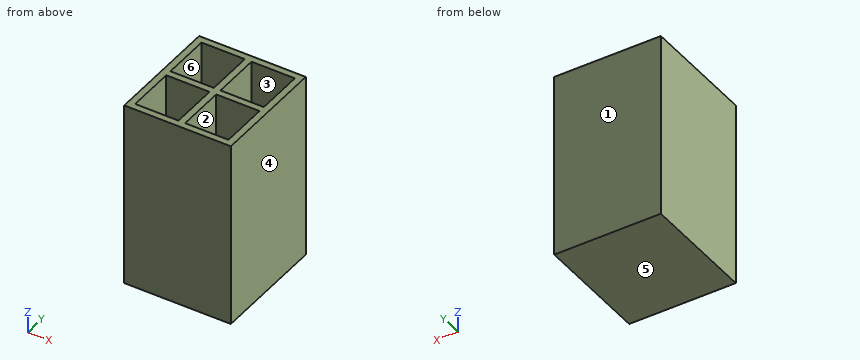
from build123d import *

# Parameters (mm, degrees)
F0_W     = 50.931696
F0_H     = 55.600882
F1_DEPTH = 88.9
F2_W     = 20.703348
F2_H     = 23.037941
F3_DEPTH = 85.852


with BuildPart() as f1:
    # F0 (on Top) → F1 (new body)
    with BuildSketch(Plane.XY):
        Rectangle(F0_W, F0_H)
    extrude(amount=F1_DEPTH)

    # F2 (on face) → F3 (cut)
    with BuildSketch(Plane.XY.offset(88.9)):
        Polygon((-22.290848, 23.611975), (-22.290848, 1.5875), (-1.5875, 1.5875), (-1.5875, 24.625441), (-20.838022, 24.625441), (-22.290848, 24.625441), align=None)
        with Locations((-11.939174, -13.10647)):
            Rectangle(F2_W, F2_H)
        with Locations((11.939174, -13.10647)):
            Rectangle(F2_W, F2_H)
        with Locations((11.939174, 13.10647)):
            Rectangle(F2_W, F2_H)
    extrude(amount=-F3_DEPTH, mode=Mode.SUBTRACT)


solid = f1.part
Work out the finished part from the listing and answer in its coordinate system (mm). Face numbers are marked on the shaded views. A direction names the side the tool comes from. Give positions to 0.01 mm unless a question says otherwise; leave off trailing zeros. Loops run counter-clockwise (first coordinate to the right, second up) from the corner with the lowest first, then second, coordinate; pieces in that order, holes last. Notation, with made-up numbers: M 79,88.5 L 133,88.5 A24 ccw 133,115.5 Z; hole C 89.5,-29 d8. An arc over 180 degrees is marked long. Use CSV: the item, a comma, the result in double quotes.
1) Determine the mould class of the marked faces 1, 2, 3 and 4 for opening direction X: released by +X, released by -X, zero draft, split by the parting line, or undercut.
Answer:
face 1,"zero draft"
face 2,"undercut"
face 3,"undercut"
face 4,"released by +X"
2) Find section B-B on x = 12. Write down the section's boundary in (y, z), plus the area to 3 significant figures.
Answer:
outline,"M -27.8,0 L 27.8,0 L 27.8,88.9 L 24.63,88.9 L 24.63,3.05 L 1.59,3.05 L 1.59,88.9 L -1.59,88.9 L -1.59,3.05 L -24.63,3.05 L -24.63,88.9 L -27.8,88.9 Z"
area,"987 mm^2"
3) Given P1, Ø10.5, axis at x = -11, y = -11.5, coming from the +Z side, flat-ended and moving along its own axis, determine where the tip first touches the part or whether it passes through.
Answer:
P1,"z = 3.05"
4) Consider L1, parallel to Y at x = 7, z = 5; L2, parallel to X at y = 23, z = 60; L3, parallel to Z at x = -16, y = 18. Determine where each line is inside the solid, lowest interval first.
Answer:
L1,"-27.8 to -24.63, -1.59 to 1.59, 24.63 to 27.8"
L2,"-25.47 to -22.29, -1.59 to 1.59, 22.29 to 25.47"
L3,"0 to 3.05"
5) Find section C-C on y = -23.5. Write down the section's boundary in (x, z).
Answer:
outline,"M -25.47,0 L 25.47,0 L 25.47,88.9 L 22.29,88.9 L 22.29,3.05 L 1.59,3.05 L 1.59,88.9 L -1.59,88.9 L -1.59,3.05 L -22.29,3.05 L -22.29,88.9 L -25.47,88.9 Z"
6) Which of the six approach directions +Z, -Z, +X, -X, +Y, -Y give full straight-line access (tool end or side, diameter ignored) to the marked faces 5 and 6?
Answer:
face 5,"-Z, +X, -X, +Y, -Y"
face 6,"+Z"
7) Find section A-A on z = 34. Write down the section's boundary in (x, y).
Answer:
outline,"M -25.47,-27.8 L 25.47,-27.8 L 25.47,27.8 L -25.47,27.8 Z; hole M -22.29,-24.63 L -1.59,-24.63 L -1.59,-1.59 L -22.29,-1.59 Z; hole M -22.29,1.59 L -1.59,1.59 L -1.59,24.63 L -22.29,24.63 Z; hole M 1.59,-24.63 L 22.29,-24.63 L 22.29,-1.59 L 1.59,-1.59 Z; hole M 1.59,1.59 L 22.29,1.59 L 22.29,24.63 L 1.59,24.63 Z"
